Can you work these out from the model? Positions are in its coordinate system, mm. A direction names the side the tool comes from. Give positions to 0.01 mm unless a question says otherwise; leave off trailing zeros. Order: outer loops, then holes, each group sorted by start corner. A loop starts at its lowest first (then second) coordinate and runs counter-clockwise, first axis right, second up. Notation, with made-up numbers: (49, -7) - (61, -7) arc R15 ccw to (61, 0) - close; hole circle Ø4 at (-2.75, 61). An arc over 180 degrees is marked (long way). One line per question, with ' | ' between items.
```python
from build123d import *

# Parameters (mm, degrees)
F0_R     = 7
F0_R_2   = 4
F1_DEPTH = 6
F2_R     = 5.5
F2_R_2   = 4
F3_DEPTH = 4
F4_R     = 7
F4_R_2   = 4
F5_DEPTH = 6
F6_SIZE  = 0.5


with BuildPart() as f1:
    # F0 (on Front) → F1 (new body)
    with BuildSketch(Plane.XZ):
        Circle(F0_R)
        Circle(F0_R_2, mode=Mode.SUBTRACT)
    extrude(amount=F1_DEPTH)

    # F2 (on face) → F3 (join)
    with BuildSketch(Plane.XZ.offset(6)):
        Circle(F2_R)
        Circle(F2_R_2, mode=Mode.SUBTRACT)
    extrude(amount=F3_DEPTH)

    # F4 (on face) → F5 (join)
    with BuildSketch(Plane.XZ.offset(10)):
        Circle(F4_R)
        Circle(F4_R_2, mode=Mode.SUBTRACT)
    extrude(amount=F5_DEPTH)

    # F6
    f6_edges = [f1.edges().sort_by_distance(p)[0] for p in [
        (-7, -6, 0),
        (-7, -10, 0),
    ]]
    chamfer(f6_edges, length=F6_SIZE)


solid = f1.part
```
(1) If I drill on line 1 (Z direction, x = 0, y = -6.25); line 2 (Z direction, x = 0, y = -12.5); line 3 (Y direction, x = -4.75, z = 3.25), over which ranges is the centre line in solid material (lowest first)?
Answer below:
line 1: -5.5 to -4, 4 to 5.5 | line 2: -7 to -4, 4 to 7 | line 3: -16 to -10, -6 to 0
(2) On a 3-axis mill with a long thin cutter (end or side, diameter ignored), from which of +Z, -Z, +X, -X, +Y, -Y can I reach the whole of each face in a straight line? I mean faces 1 (the face through (-5, -10, 3)), 2 (the face through (6.466, -2.712, -2.681)). Say none if no direction works.
Answer below:
face 1: none | face 2: +Y, -Y
(3) Imagine slicing it at C-C (y = -12.75). List the corners of the cut face in (x, z) for me.
Answer below:
outline: circle Ø14 at (0, 0); hole circle Ø8 at (0, 0)
(4) If we mould it in two halves opening along X, with no side actions, what happens to faces 3 (the face through (-1.19, -7.97, -5.37)), 4 (the face through (-0.867, -7.888, -3.905)), 5 (the face through (-5, -6, 3))? For each: released by +X, released by -X, zero draft, split by the parting line, or undercut.
Answer below:
face 3: split by the parting line | face 4: undercut | face 5: zero draft
(5) Imagine slicing it at B-B (y = -6.75). List the corners of the cut face in (x, z) for me, and give its area (3 significant figures).
Answer below:
outline: circle Ø11 at (0, 0); hole circle Ø8 at (0, 0) | area: 44.8 mm^2
(6) Will these pins go through, and if not, where does the flat tip stop? pin 1 (6 mm diameter, centred on x = 5, y = -9.5, fed in from +Z); pin 2 (6 mm diameter, centred on x = 5, y = -2, fed in from +Z); pin 3 (1.5 mm diameter, centred on x = -4.5, y = -9, fed in from +Z).
Answer below:
pin 1: z = 6.65 | pin 2: z = 6.71 | pin 3: z = 4.02
(7) Imagine slicing it at A-A (x = 0). List the corners of the cut face in (y, z) for me, and give its area (3 significant figures).
Answer below:
outline: (-16, -7) - (-10.5, -7) - (-10, -6.5) - (-10, -5.5) - (-6, -5.5) - (-6, -6.5) - (-5.5, -7) - (0, -7) - (0, -4) - (-16, -4) - close; (-16, 4) - (0, 4) - (0, 7) - (-5.5, 7) - (-6, 6.5) - (-6, 5.5) - (-10, 5.5) - (-10, 6.5) - (-10.5, 7) - (-16, 7) - close | area: 83.5 mm^2
